Work out the finished part from the listing and answer in its coordinate system (mm). Face numbers are marked on the shaded views. A direction names the side the tool comes from. Round coordinates to 2 decimals unless told otherwise and drop trailing zeros. Write each loop counter-clockwise with the first axis right and the second up, starting at its lowest first coordinate (ties: lowest second). Pieces come first, ordered by that corner, then holes. Notation, with made-up numbers: M 82,47 L 86,47 A15 cw 86,75 Z; hole C 59,-24.75 d10. An arc over 180 degrees is marked long. One line per item, written item: value. Start each with the question number.
Q1. Find section D-D (x = -263). Write down the section's boundary in (y, z), and give its area (3 significant figures).
Q2. Given pin 1 Ø1.5 at (x, z) = (-145, 85) entering from +Y; pin 2 Ø6 at (x, z) = (-313.73, 142.56) entering from +Y; pin 3 Ø23 at (y, z) = (23.02, 190.86) entering from +X, each flat-ended and moving along its own axis, determine where each tip first touches the part or whether it passes through.
Q3. The mould has two halves that part along Z. Classify the marked faces 6, 7 and 8: released by +Z, released by -Z, zero draft, split by the parting line, or undercut.
Q4. Find section B-B (z = 216). Write down the section's boundary in (x, y), and give its area (3 significant figures).
Q5. Find section A-A (x = -189.5). Write down the section's boundary in (y, z).
Q6. A tool of negligible diameter and unlimited length cuts with its end or side. For the marked faces 1, 2, 3, 4 and 5, from which of +Z, -Z, +X, -X, +Y, -Y can it reach the whole face along a straight path? Write none if from no direction.
Q7. Find section C-C (y = -71). Write down the section's boundary in (x, z), and give its area (3 significant figures).
Q8. Consider probe 1 along Y at (x, z) = (-144.5, 139); probe 2 along Z at (x, y) = (-53.5, 27); probe 3 along Y at (x, z) = (-360, 155.5). Determine where each line is inside the solid, lowest interval first.
Autodesk Inventor part; units mm, degrees
ref_plane "YZ Plane" through (0, 0, 0) normal (1, 0, 0) x (0, 1, 0)
ref_plane "XZ Plane" through (0, 0, 0) normal (0, 1, 0) x (-1, 0, 0)
ref_plane "XY Plane" through (0, 0, 0) normal (0, 0, 1) x (1, 0, 0)
sketch "Sketch1" plane through (0, 0, 0) normal (1, 0, 0) x (0, 1, 0)
  line L0 (10.5163, 293.3597) -> (7.5163, 293.3597)
  line L1 (7.5163, 293.3597) -> (7.5163, 43.3597)
  line L2 (7.5163, 43.3597) -> (10.5163, 43.3597)
  line L3 (10.5163, 43.3597) -> (10.5163, 293.3597)
  line L4 (10.5163, 293.3597) -> (7.5163, 43.3597) construction
  line L5 (7.5163, 293.3597) -> (10.5163, 43.3597) construction
  line L6 (7.5163, 46.3597) -> (-192.4837, 46.3597)
  line L7 (-192.4837, 46.3597) -> (-192.4837, 43.3597)
  line L8 (-192.4837, 43.3597) -> (7.5163, 43.3597)
  line L9 (7.5163, 43.3597) -> (7.5163, 46.3597)
  line L10 (7.5163, 46.3597) -> (-192.4837, 43.3597) construction
  line L11 (-192.4837, 46.3597) -> (7.5163, 43.3597) construction
  line L12 (7.5163, 168.3597) -> (-42.4837, 168.3597)
  line L13 (7.5163, 168.3597) -> (57.5163, 168.3597) construction
  line L14 (7.5163, 290.3597) -> (-192.4837, 290.3597)
  line L15 (-192.4837, 290.3597) -> (-192.4837, 293.3597)
  line L16 (-192.4837, 293.3597) -> (7.5163, 293.3597)
  line L17 (7.5163, 290.3597) -> (-192.4837, 293.3597) construction
  line L18 (-192.4837, 290.3597) -> (7.5163, 293.3597) construction
  line L19 (-189.4837, 290.3597) -> (-192.4837, 290.3597)
  line L20 (-192.4837, 290.3597) -> (-192.4837, 46.3597)
  line L21 (-192.4837, 46.3597) -> (-189.4837, 46.3597)
  line L22 (-189.4837, 46.3597) -> (-189.4837, 290.3597)
  line L23 (-189.4837, 290.3597) -> (-192.4837, 46.3597) construction
  line L24 (-192.4837, 290.3597) -> (-189.4837, 46.3597) construction
  point P0 (0, 0)
  point P1 (9.0163, 168.3597)
  point P2 (-92.4837, 44.8597)
  point P3 (-92.4837, 291.8597)
  point P4 (-189.2359, -83.872)
  point P5 (7.5163, 290.3597)
  point P6 (7.5163, 46.3597)
  point P7 (-190.9837, 168.3597)
  point P8 (-189.4837, 46.3597)
  point P9 (-189.4837, 290.3597)
  dimension "d0" = 3
  dimension "d1" = 250
  dimension "d2" = 200
  dimension "d3" = 3
  dimension "d4" = 50
  dimension "d5" = 180
  dimension "d19" = 244
extrude "Extrusion1" add sketch "Sketch1" against normal blind 200 contours L3 L2 L1 L0 | L1 L14 L15 L16 | L8 L7 L6 L1 | L22 L6 L20 L14
sketch "Sketch3" plane through (-200, 0, 0) normal (-1, 0, 0) x (0, 0, 1)
  line L0 (43.3597, -189.4837) -> (293.3597, -189.4837)
  line L1 (293.3597, -189.4837) -> (293.3597, -192.4837)
  line L2 (293.3597, -192.4837) -> (43.3597, -192.4837)
  line L3 (43.3597, -192.4837) -> (43.3597, -189.4837)
  line L4 (43.3597, -189.4837) -> (293.3597, -192.4837) construction
  line L5 (293.3597, -189.4837) -> (43.3597, -192.4837) construction
  line L6 (46.3597, -189.4837) -> (290.3597, -189.4837)
  line L7 (290.3597, -189.4837) -> (46.3597, -189.4837)
  line L8 (290.3597, -189.4837) -> (534.3597, -189.4837) construction
  point P0 (0, 0)
  point P1 (168.3597, -190.9837)
  point P2 (168.3597, -189.4837)
  dimension "d20" = 250
  dimension "d21" = 3
  dimension "d22" = 244
  dimension "d23" = 180
extrude "Extrusion3" add sketch "Sketch3" along normal blind 220
sketch "Sketch7" plane through (0, -189.4837, 290.3597) normal (0, 1, 0) x (1, 0, 0)
  line L0 (-200, 247) -> (-420, 247)
  line L1 (-200, -3) -> (-420, -3)
  line L2 (-420, -3) -> (-420, 247)
  point P0 (0, 290.3597)
  point P1 (-355, 97)
  point P2 (-355, 147.8)
  point P3 (-313.725, 147.8)
  point P4 (-313.725, 97)
  point P5 (-200, 244)
  point P6 (-200, 0)
  point P7 (-350, 369)
  point P8 (-350, -125)
  dimension "d53" = 50.8
  dimension "d54" = 50.8
  dimension "d55" = 41.275
  dimension "d56" = 41.275
  dimension "d59" = 100
  dimension "d60" = 100
  dimension "d61" = 65
  dimension "d62" = 65
hole "Hole1" at (-355, -189.4837, 193.3597) at (-355, -189.4837, 142.5597) at (-313.725, -189.4837, 142.5597) at (-313.725, -189.4837, 193.3597) direction (0, -1, 0) diameter 4.572 depth 26 tip angle 118
sketch "Sketch8" plane through (0, 10.5163, 293.3597) normal (0, 1, 0) x (1, 0, 0)
  line L0 (-3, 250) -> (0, 250)
  line L1 (0, 250) -> (0, 0)
  line L2 (0, 0) -> (-3, 0)
  line L3 (-3, 0) -> (-3, 250)
  line L4 (-3, 250) -> (0, 0) construction
  line L5 (0, 250) -> (-3, 0) construction
  line L6 (0, 250) -> (0, 0)
  line L7 (-200, 250) -> (-3, 250)
  line L8 (-3, 250) -> (-3, 247)
  line L9 (-3, 247) -> (-200, 247)
  line L10 (-200, 247) -> (-200, 250)
  line L11 (-200, 250) -> (-3, 247) construction
  line L12 (-3, 250) -> (-200, 247) construction
  line L13 (-200, 3) -> (-3, 3)
  line L14 (-3, 3) -> (-3, 0)
  line L15 (-3, 0) -> (-200, 0)
  line L16 (-200, 0) -> (-200, 3)
  line L17 (-200, 3) -> (-3, 0) construction
  line L18 (-3, 3) -> (-200, 0) construction
  point P0 (0, 293.3597)
  point P1 (-1.5, 125)
  point P2 (0, 125)
  point P3 (-101.5, 248.5)
  point P4 (-101.5, 1.5)
  point P5 (-3, 3)
  dimension "d63" = 3
  dimension "d64" = 250
  dimension "d82" = 197
  dimension "d83" = 3
  dimension "d84" = 197
  dimension "d85" = 3
extrude "Extrusion7" add sketch "Sketch8" along normal blind 65 contours L0 L1 L2 L3
sketch "Sketch9" plane through (0, 0, 0) normal (1, 0, 0) x (0, 0, -1)
  line L0 (-293.3597, 10.5163) -> (-43.3597, 10.5163)
  line L1 (-293.3597, 75.5163) -> (-293.3597, -192.4837)
  point P0 (0, 0)
  point P1 (-235.8597, 23.0163)
  point P2 (-190.8597, 23.0163)
  point P3 (-145.8597, 23.0163)
  point P4 (-100.8597, 23.0163)
  dimension "d74" = 12.5
  dimension "d75" = 12.5
  dimension "d76" = 12.5
  dimension "d77" = 12.5
  dimension "d78" = 45
  dimension "d79" = 45
  dimension "d80" = 45
  dimension "d81" = 57.5
hole "Hole2" at (0, 23.0163, 235.8597) at (0, 23.0163, 190.8597) at (0, 23.0163, 145.8597) at (0, 23.0163, 100.8597) direction (-1, 0, 0) diameter 20 depth 26 tip angle 118
extrude "Extrusion8" add sketch "Sketch8" along normal blind 65 contours L3 L9 L10 L7 | L3 L15 L16 L13
sketch "Sketch10" plane through (0, -189.4837, 290.3597) normal (0, 1, 0) x (1, 0, 0)
  line L0 (-3, 0) -> (0, 0)
  line L1 (0, 0) -> (0, 244)
  line L2 (0, 244) -> (-3, 244)
  line L3 (-3, 244) -> (-3, 0)
  line L4 (-3, 0) -> (0, 244) construction
  line L5 (0, 0) -> (-3, 244) construction
  line L6 (0, 244) -> (0, 0)
  point P0 (0, 290.3597)
  point P1 (-1.5, 122)
  point P2 (0, 122)
  dimension "d89" = 3
  dimension "d90" = 244
extrude "Extrusion9" add sketch "Sketch10" along normal blind 65
sketch "Sketch11" plane through (0, 0, 0) normal (1, 0, 0) x (0, 0, -1)
  line L0 (-290.3597, -189.4837) -> (-46.3597, -189.4837)
  line L1 (-293.3597, 75.5163) -> (-293.3597, -192.4837)
  point P0 (0, 0)
  point P1 (-235.8597, -176.9837)
  point P2 (-190.8597, -176.9837)
  point P3 (-145.8597, -176.9837)
  point P4 (-100.8597, -176.9837)
  dimension "d100" = 12.5
  dimension "d101" = 12.5
  dimension "d102" = 12.5
  dimension "d103" = 12.5
  dimension "d104" = 57.5
  dimension "d105" = 45
  dimension "d106" = 45
  dimension "d107" = 45
hole "Hole3" at (0, -176.9837, 235.8597) at (0, -176.9837, 190.8597) at (0, -176.9837, 145.8597) at (0, -176.9837, 100.8597) direction (-1, 0, 0) diameter 20 depth 26 tip angle 118
properties part number "Valves_Pump Holder"
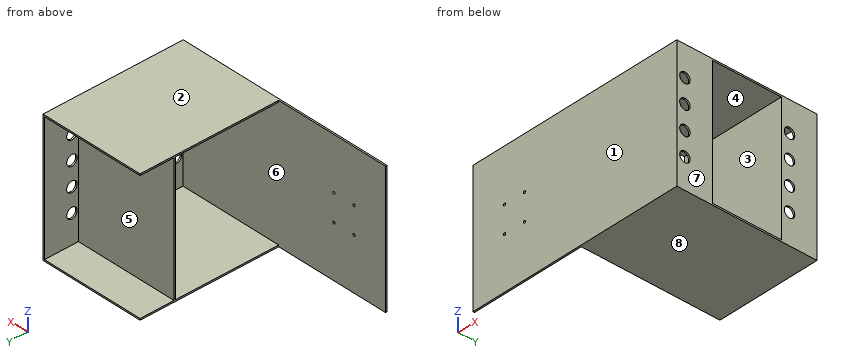
The answers:
1. outline: M -192.48,43.36 L -189.48,43.36 L -189.48,293.36 L -192.48,293.36 Z
1. area: 750 mm2
2. pin 1: y = 10.52
2. pin 2: y = -189.48
2. pin 3: x = 0
3. face 6: undercut
3. face 7: zero draft
3. face 8: released by -Z
4. outline: M -420,-192.48 L 0,-192.48 L 0,-124.48 L -3,-124.48 L -3,-189.48 L -420,-189.48 Z; M -200,7.52 L 0,7.52 L 0,75.52 L -3,75.52 L -3,10.52 L -200,10.52 Z
4. area: 2,250 mm2
5. outline: M -192.48,43.36 L 75.52,43.36 L 75.52,46.36 L 10.52,46.36 L 10.52,290.36 L 75.52,290.36 L 75.52,293.36 L -192.48,293.36 Z; hole M -189.48,46.36 L 7.52,46.36 L 7.52,290.36 L -189.48,290.36 Z
6. face 1: +Z, -Z, +X, -X, -Y
6. face 2: +Z, +X, -X, +Y, -Y
6. face 3: +X, -X
6. face 4: -X
6. face 5: -X, +Y
7. outline: M -200,43.36 L 0,43.36 L 0,46.36 L -200,46.36 Z; M -200,290.36 L 0,290.36 L 0,293.36 L -200,293.36 Z
7. area: 1,200 mm2
8. probe 1: -192.48 to -189.48, 7.52 to 10.52
8. probe 2: 43.36 to 46.36, 290.36 to 293.36
8. probe 3: -192.48 to -189.48
